Part model, mm, in its own coordinate system. A direction names the side the tool comes from. Coordinates: 2 decimals unless noted, no trailing zeros. Loops run counter-clockwise (first coordinate to the right, second up) from the corner with the lowest first, then second, coordinate; pieces in that order, holes last. Notation, with made-up numbers: (53, -26) - (88, -26) arc R20 cw to (88, 7) - close; hole circle Ø2 at (19.5, 14). An arc over 180 degrees is marked (long way). Answer as CSV lines item,"result".
from build123d import *

# Parameters (mm, degrees)
F1_DEPTH = 25.4
F2_W     = 25.4
F2_H     = 7.62
F3_DEPTH = 19.05
F5_DEPTH = 19.05
F6_R     = 5.08
F7_DEPTH = 3.175
F8_DEPTH = 3.175
F9_R     = 3.175
F10_SIZE = 0.762


with BuildPart() as f1:
    # F0 (on Top) → F1 (new body)
    with BuildSketch(Plane.XY):
        with BuildLine():
            Line((25.4, 15.875), (12.7, 15.875))
            ThreePointArc((12.7, 15.875), (0, 3.175), (-12.7, 15.875))
            Line((-12.7, 15.875), (-25.4, 15.875))
            Line((-25.4, 15.875), (-25.4, -15.875))
            Line((-25.4, -15.875), (25.4, -15.875))
            Line((25.4, -15.875), (25.4, 15.875))
        make_face()
    extrude(amount=F1_DEPTH)

    # F2 (on face) → F3 (cut)
    with BuildSketch(Plane.XY.offset(25.4)):
        with Locations((0, -12.065)):
            Rectangle(F2_W, F2_H)
    extrude(amount=-F3_DEPTH, mode=Mode.SUBTRACT)

    # F4 (on face) → F5 (cut)
    with BuildSketch(Plane.XY.offset(25.4)):
        Polygon((-25.4, 15.875), (-25.4, -15.875), (-16.51, -15.875), (-16.51, 0), (-13.97, 0), (-13.97, 15.875), align=None)
        Polygon((25.4, 15.875), (13.97, 15.875), (13.97, 0), (16.51, 0), (16.51, -15.875), (25.4, -15.875), align=None)
    extrude(amount=-F5_DEPTH, mode=Mode.SUBTRACT)

    # F6
    f6_edges = [f1.edges().sort_by_distance(p)[0] for p in [
        (25.4, 15.875, 3.175),
        (-25.4, 15.875, 3.175),
    ]]
    fillet(f6_edges, radius=F6_R)

    # F7 (add): a face of the model
    f7_faces = [f1.faces().sort_by_distance(p)[0] for p in [
        (16.51, -7.9375, 15.875),
    ]]
    extrude(f7_faces, amount=F7_DEPTH)

    # F8 (add): a face of the model
    f8_faces = [f1.faces().sort_by_distance(p)[0] for p in [
        (-16.51, -7.9375, 15.875),
    ]]
    extrude(f8_faces, amount=F8_DEPTH)

    # F9
    f9_edges = [f1.edges().sort_by_distance(p)[0] for p in [
        (-13.97, 0, 15.875),
        (13.97, 0, 15.875),
    ]]
    fillet(f9_edges, radius=F9_R)

    # F10
    f10_edges = [f1.edges().sort_by_distance(p)[0] for p in [
        (0, -8.255, 25.4),
        (12.7, -12.065, 25.4),
        (-12.7, -12.065, 25.4),
        (0, 3.175, 25.4),
    ]]
    chamfer(f10_edges, length=F10_SIZE)


solid = f1.part
Q1. Wall check: L1, parallel to X at y = -13.5, z = 20 (3 decimals); L2, parallel to Z at x = 20, y = -2.5; L3, parallel to X at y = -4.5, z = 19 (3 decimals). Give the ranges that are in metal, low to high.
Results:
L1,"x = -19.685 to -12.7, 12.7 to 19.685"
L2,"z = 0 to 6.35"
L3,"x = -19.685 to 19.685"
Q2. Saw through at A-A (x = 0). Give the cut face in (y, z) (3 decimals), then the cut area to 3 significant figures.
Results:
outline,"(-15.875, 0) - (3.175, 0) - (3.175, 24.638) - (2.413, 25.4) - (-7.493, 25.4) - (-8.255, 24.638) - (-8.255, 6.35) - (-15.875, 6.35) - close"
area,"338 mm^2"
Q3. Saw through at C-C (z = 10.25). Give the cut face in (x, y) (3 decimals), then the cut area to 3 significant figures.
Results:
outline,"(-19.685, -15.875) - (-12.7, -15.875) - (-12.7, -8.255) - (12.7, -8.255) - (12.7, -15.875) - (19.685, -15.875) - (19.685, 0) - (17.145, 0) arc R3.175 cw to (13.97, 3.175) - (13.97, 15.875) - (12.7, 15.875) arc R12.7 cw to (-12.7, 15.875) - (-13.97, 15.875) - (-13.97, 3.175) arc R3.175 cw to (-17.145, 0) - (-19.685, 0) - close"
area,"626 mm^2"
Q4. Which spindle directions (+Z, -Z, +X, -X, +Y, -Y) get a long thin tool onto all of the face, cutting with end or side? Do faces 1 (the face through (12.7, -12, 16)), 2 (the face through (-23.9, 14.4, 3.2)), 3 (the face through (-14.88, 0.95, 15.74)), 4 (the face through (14.92, 0.91, 15.74)), 5 (the face through (-19.685, -8, 16)). Say none if no direction does.
Results:
face 1,"+Z, -Y"
face 2,"+Z, -Z, -X, +Y"
face 3,"+Z, -X, +Y"
face 4,"+Z, +X, +Y"
face 5,"+Z, -X, +Y, -Y"
Q5. Flat gauge pins, fed straight in: pin 1 (6 mm diameter, centred on y = -13.5, z = 13, fed in from +X) (3 decimals); pin 2 (3 mm diameter, centred on x = -2, z = 12.5, fed in from -Y) (3 decimals); pin 3 (1.3 mm diameter, centred on x = 19, z = 12, fed in from +Y); pin 4 (12 mm diameter, centred on x = 8, z = 18, fed in from +Y) (3 decimals). Where does each tip first touch, or does it go through?
Results:
pin 1,"stops at x = 19.685"
pin 2,"stops at y = -8.255"
pin 3,"stops at y = 0"
pin 4,"stops at y = 15.875"
Q6. Two-plate mould, pull along X, no slides. Class faces 6 (the face through (13.97, 10, 16)), 7 (the face through (0, -8.255, 16)), 8 (the face through (-13, 15.875, 7)): released by +X, released by -X, zero draft, split by the parting line, or undercut.
Results:
face 6,"released by +X"
face 7,"undercut"
face 8,"zero draft"
Q7. Saw through at D-D (z = 2.25). Give the cut face in (x, y) (3 decimals), then the cut area to 3 significant figures.
Results:
outline,"(-25.4, -15.875) - (25.4, -15.875) - (25.4, 10.795) arc R5.08 ccw to (20.32, 15.875) - (12.7, 15.875) arc R12.7 cw to (-12.7, 15.875) - (-20.32, 15.875) arc R5.08 ccw to (-25.4, 10.795) - close"
area,"1,350 mm^2"
Q8. Saw through at B-B (y = -13). Give the cut face in (x, z) (3 decimals).
Results:
outline,"(-25.4, 0) - (25.4, 0) - (25.4, 6.35) - (19.685, 6.35) - (19.685, 25.4) - (13.462, 25.4) - (12.7, 24.638) - (12.7, 6.35) - (-12.7, 6.35) - (-12.7, 24.638) - (-13.462, 25.4) - (-19.685, 25.4) - (-19.685, 6.35) - (-25.4, 6.35) - close"
